Model file for the job. Use its own axes, mm. A direction names the side the tool comes from. Coordinates: 2 decimals unless noted, no trailing zeros. Loops run counter-clockwise (first coordinate to the right, second up) from the corner with the lowest first, then second, coordinate; pieces in that order, holes last. Notation, with made-up numbers: (-31.5, 32) -> (15.5, 32) arc R29 cw to (15.5, 64) -> close; hole circle Ø3 at (-38.75, 10). An arc over 180 degrees is marked (long way). Use one line per item in the form item = value.
```python
from build123d import *

# Parameters (mm, degrees)
F0_W           = 15
F0_H           = 6.35
F1_DEPTH       = 6.35
F2_R           = 2
F5_D           = 2.05
F5_DEPTH       = 6
F5_TIP         = 0.6158821345
F5_ON_F3_D     = 2.05
F5_ON_F3_DEPTH = 6
F5_ON_F3_TIP   = 0.6158821345
F6_D           = 2.5
F6_CSINK_D     = 4.7
F6_CSINK_ANGLE = 90
F7_D           = 2
F7_DEPTH       = 8
F7_TIP         = 0.600860619


# Not quite as in the source:
# - a length typed as a fraction of an inch, garbled in the dataset ("3 / 203.2 mm" for 3/8 in), is restored


with BuildPart() as f1:
    # F0 (on Top) → F1 (new body)
    with BuildSketch(Plane.XY):
        Polygon((15, 15), (-15, 15), (-15, -20), (-7.5, -20), (7.5, -20), (15, -20), align=None)
        with BuildLine():
            ThreePointArc((0, 11.4), (8.0610173055, 8.0610173055), (11.4, 0))
            ThreePointArc((11.4, 0), (-8.0610173055, -8.0610173055), (0, 11.4))
        make_face(mode=Mode.SUBTRACT)
        with Locations((0, -23.175)):
            Rectangle(F0_W, F0_H)
    extrude(amount=F1_DEPTH)

    # F2
    f2_edges = [f1.edges().sort_by_distance(p)[0] for p in [
        (15, 15, 3.175),
        (-15, 15, 3.175),
    ]]
    fillet(f2_edges, radius=F2_R)

    # F5
    with Locations(Plane.XZ.offset(20)):
        with Locations((-11.25, 3.175)):
            Hole(F5_D / 2, depth=F5_DEPTH)
            with Locations((0, 0, -(F5_DEPTH + F5_TIP / 2))):  # 118° drill point
                Cone(0, F5_D / 2, F5_TIP, mode=Mode.SUBTRACT)

    # F5 on F3
    with Locations(Plane.XZ.offset(20)):
        with Locations((11.25, 3.175)):
            Hole(F5_ON_F3_D / 2, depth=F5_ON_F3_DEPTH)
            with Locations((0, 0, -(F5_ON_F3_DEPTH + F5_ON_F3_TIP / 2))):  # 118° drill point
                Cone(0, F5_ON_F3_D / 2, F5_ON_F3_TIP, mode=Mode.SUBTRACT)

    # F6 (through all)
    with Locations(Plane(origin=(0, 0, 0), x_dir=(1, 0, 0), z_dir=(0, 0, -1))):
        with Locations((-11.5, -11.5), (11.5, -11.5), (-11.5, 11.5), (11.5, 11.5), (0, 23.175)):
            CounterSinkHole(F6_D / 2, F6_CSINK_D / 2, counter_sink_angle=F6_CSINK_ANGLE)

    # F7
    with Locations(Plane(origin=(0, 0, 0), x_dir=(1, 0, 0), z_dir=(0, 0, -1))):
        with Locations((13.2, 0), (0, -13.2), (-13.2, 0), (0, 15.7)):
            Hole(F7_D / 2, depth=F7_DEPTH)
            with Locations((0, 0, -(F7_DEPTH + F7_TIP / 2))):  # 118° drill point
                Cone(0, F7_D / 2, F7_TIP, mode=Mode.SUBTRACT)


solid = f1.part
```
Q1. Wall check: line 1 along Y through (x, z) = (0, 1.5) (3 decimals); line 2 along Y through (x, z) = (11.5, 4.25); line 3 along X through (y, z) = (5, 2.25) (3 decimals). Give the ranges that are in metal, low to high.
Result:
line_1 = -26.35 to -24.425, -21.925 to -16.7, -14.7 to -11.4, 11.4 to 12.2, 14.2 to 15
line_2 = -20 to -12.75, -10.25 to 10.25, 12.75 to 15
line_3 = -15 to -10.245, 10.245 to 15
Q2. Band-saw the part on D-D, the plane z = 5. State how many separate pieces and enclosed holes the cut face has, and give its area (3 significant figures).
Result:
separate_pieces = 1
enclosed_holes = 10
area = 698 mm2
Q3. Band-saw the part on A-A, the plane y = -15.7. Write the cut outline in (x, z) (3 decimals).
Result:
outline = (-15, 0) -> (-1, 0) -> (-1, 6.35) -> (-15, 6.35) -> close; (1, 0) -> (15, 0) -> (15, 6.35) -> (1, 6.35) -> close; hole circle Ø2.05 at (-11.25, 3.175); hole circle Ø2.05 at (11.25, 3.175)
Q4. Band-saw the part on B-B, the plane x = -8. Write the cut outline in (y, z).
Result:
outline = (-20, 0) -> (-8.12, 0) -> (-8.12, 6.35) -> (-20, 6.35) -> close; (8.12, 0) -> (15, 0) -> (15, 6.35) -> (8.12, 6.35) -> close
Q5. Mould opens along Z. For faces 4 (the face through (-0.46, 14.09, 3.22)), 5 (the face through (-7, -10, 0)), 6 (the face through (-11.43, -13.49, 3.18)), 7 (the face through (12.005, -16.958, 3.868)) say: released by +Z, released by -Z, zero draft, split by the parting line, or undercut.
Result:
face_4 = zero draft
face_5 = released by -Z
face_6 = undercut
face_7 = undercut
Q6. Which spindle directions (+Z, -Z, +X, -X, +Y, -Y) get a long thin tool onto all of the face, cutting with end or side? Do faces 1 (the face through (0.217, -14.724, 3.219)), 2 (the face through (-10.495, -16.958, 3.868)), 3 (the face through (7.5, -23, 3)). Say none if no direction does.
Result:
face_1 = +Z, -Z
face_2 = -Y
face_3 = +Z, -Z, +X, -Y
Q7. Pin check, flat tips, straight feed: pin 1 Ø2 at (x, y) = (9.5, -11.5) entering from -Z; pin 2 Ø2.5 at (x, z) = (-11.25, 3.175) entering from -Y; pin 3 Ø3 at (y, z) = (-24, 2) entering from +X; pin 4 Ø4 at (x, y) = (-11.5, -11.5) entering from -Z. Stop position of each tip, or through.
Result:
pin_1 = 0
pin_2 = -20
pin_3 = 7.5
pin_4 = 0.35
Q8. Band-saw the part on C-C, the plane y = 7. Write the cut outline in (x, z).
Result:
outline = (-15, 0) -> (-9, 0) -> (-9, 6.35) -> (-15, 6.35) -> close; (9, 0) -> (15, 0) -> (15, 6.35) -> (9, 6.35) -> close
